For this review, take the finished solid that the model builds, in its own axes (mm). A direction names the side the tool comes from. Give positions to 0.01 mm unless a question says otherwise; leave off trailing zeros. Order: outer loops, then holes, each group sorted by start corner. A loop starts at its lowest first (then second) coordinate and runs counter-clockwise, first axis right, second up.
from build123d import *

# Parameters (mm, degrees)
ESQUISSE1_R        = 8
BOSS_EXTRU_1_DEPTH = 5
CONG_1_R           = 10


with BuildPart() as part:
    # Esquisse1 → Boss.-Extru.1 (new body)
    with BuildSketch(Plane(origin=(0, 0, 0), x_dir=(1, 0, 0), z_dir=(0, 1, 0))):
        Polygon((40, -7.5), (45, -7.5), (45, -17.5), (40, -17.5), (40, -25), (0, -25), (0, 0), (40, 0), align=None)
        with Locations((12.5, -12.5)):
            Circle(ESQUISSE1_R, mode=Mode.SUBTRACT)
    extrude(amount=BOSS_EXTRU_1_DEPTH)

    # Congé1
    cong_1_edges = [part.edges().sort_by_distance(p)[0] for p in [
        (0, 2.5, 0),
        (0, 2.5, 25),
    ]]
    fillet(cong_1_edges, radius=CONG_1_R)


solid = part.part
1) Clearance check with flat-ended pins moving along their axes: pin 1 (2 mm diameter, centred on y = 0.5, z = 20.5, fed in from +X); pin 2 (1 mm diameter, centred on y = 3, z = 8, fed in from -X); pin 3 (2.5 mm diameter, centred on x = 42, y = 1.5, fed in from +Z). State where each tip first meets the part, or that it passes through.
Answer sheet:
pin 1: stops at x = 40
pin 2: stops at x = 0.11
pin 3: stops at z = 17.5
2) Tool access review of faces 4 (the face through (23, 0, 12)), 5 (the face through (43, 2, 17.5)), 6 (the face through (42, 2, 7.5)): name each direction out of +Z, -Z, +X, -X, +Y, -Y from which nothing blocks a thin tool from reaching the whole face with its end or side.
Answer sheet:
face 4: +Z, -Z, +X, -X, -Y
face 5: +Z, +X, +Y, -Y
face 6: -Z, +X, +Y, -Y
3) We need section D-D on z = 4. Give the boundary of the cut face in (x, y).
Answer sheet:
outline: (2, 0) - (40, 0) - (40, 5) - (2, 5) - close
4) Draft analysis for pull direction X (two halves, no side actions). For faces 1 (the face through (45, 2, 12)), 2 (the face through (10.77, 2.46, 20.31)), 3 (the face through (3.01, 2.54, 2.85)), state which applies: +X half, -X half, draft (parallel to the pull), parting line (faces both ways), or undercut.
Answer sheet:
face 1: +X half
face 2: undercut
face 3: -X half
5) We need section B-B on x = 12.5. Give the boundary of the cut face in (y, z).
Answer sheet:
outline: (0, 0) - (5, 0) - (5, 4.5) - (0, 4.5) - close; (0, 20.5) - (5, 20.5) - (5, 25) - (0, 25) - close
6) We need section C-C on z = 13.5. Give the boundary of the cut face in (x, y), then the cut area to 3 significant figures.
Answer sheet:
outline: (0, 0) - (4.56, 0) - (4.56, 5) - (0, 5) - close; (20.44, 0) - (45, 0) - (45, 5) - (20.44, 5) - close
area: 146 mm2
7) We need section A-A on y = 1.1. Give the boundary of the cut face in (x, z).
Answer sheet:
outline: (0, 10) arc R10 ccw to (10, 0) - (40, 0) - (40, 7.5) - (45, 7.5) - (45, 17.5) - (40, 17.5) - (40, 25) - (10, 25) arc R10 ccw to (0, 15) - close; hole circle Ø16 at (12.5, 12.5)
8) To check wall thickness, follow line 1 (Z direction, x = 12.5, y = 2.45); line 2 (X direction, y = 2.7, z = 12.5); line 3 (Z direction, x = 11, y = 0.8). State the ranges of each line that lie inside material, in increasing order.
Answer sheet:
line 1: z = 0 to 4.5, 20.5 to 25
line 2: x = 0 to 4.5, 20.5 to 45
line 3: z = 0 to 4.64, 20.36 to 25
